Input: dimensioned drawing with shaded views. Units: mm. Origin: part minimum x, y, z. Coordinates: 2 decimals unless noted, no trailing zeros. Order: outer loops, then holes, each group sorted by start corner. A loop starts at its lowest first (then second) coordinate and runs counter-clockwise, first axis right, second up. Notation, with made-up numbers: (72.5, -14.5) - (120.5, -14.5) arc R16 cw to (120.5, 15.5) - close; hole circle Ø3 at (-39.5, -8). An arc over 180 degrees is marked (long way). Answer as CSV lines item,"result". Start each with the question number.
Item 1: Material intervals for line 1 along Z through (x, y) = (80, 1.2); line 2 along X through (y, z) = (0.9, 115); line 3 along X through (y, z) = (3.2, 25), sorted ascending.
Item 2: Section C-C (z = 109.5). Output: boundary loops of the cut face in (x, y).
Item 3: Section B-B (x = 175). Output: boundary loops of the cut face in (y, z).
Item 4: Section A-A (y = 1.7). State how many separate pieces and enclosed holes the cut face has, and give its area (3 significant figures).
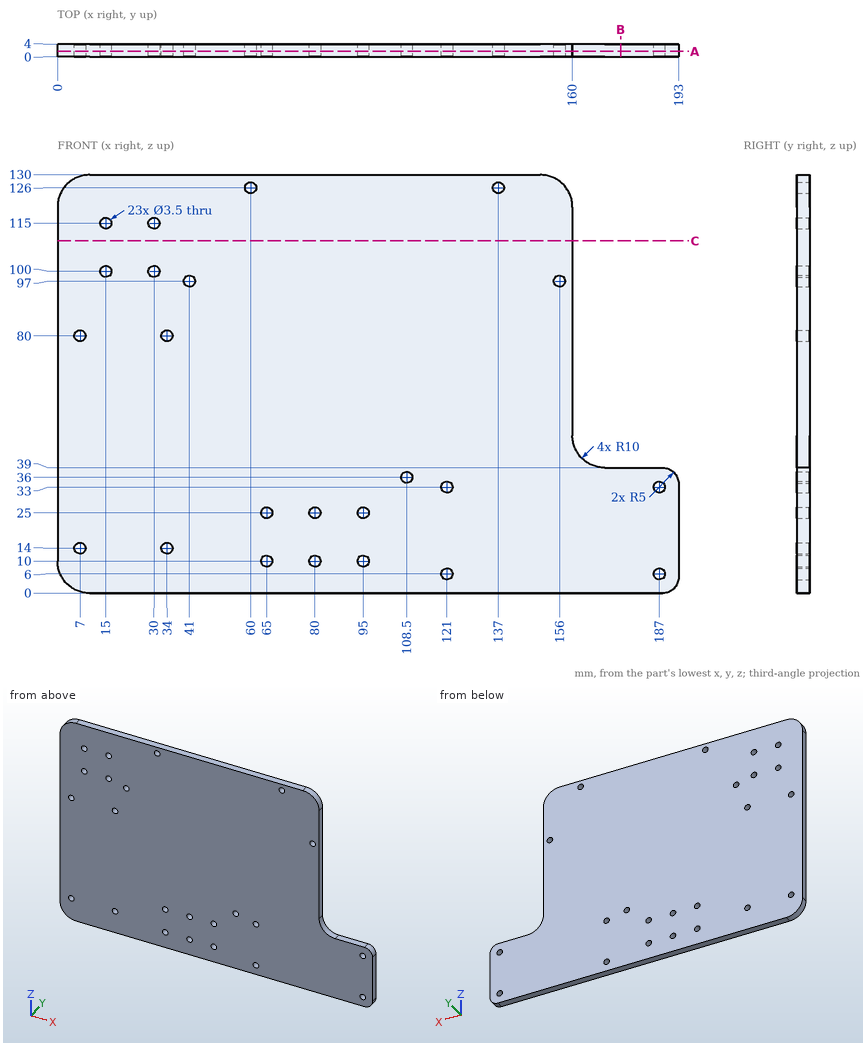
Determined:
1,line 1,"z = 0 to 8.25, 11.75 to 23.25, 26.75 to 130"
1,line 2,"x = 0 to 13.25, 16.75 to 28.25, 31.75 to 160"
1,line 3,"x = 0 to 63.25, 66.75 to 78.25, 81.75 to 93.25, 96.75 to 193"
2,outline,"(0, 0) - (160, 0) - (160, 4) - (0, 4) - close"
3,outline,"(0, 0) - (4, 0) - (4, 39) - (0, 39) - close"
4,separate pieces,"1"
4,enclosed holes,"23"
4,area,"21,800 mm^2"
